```python
from build123d import *

# Parameters (mm, degrees)
SKETCH1_W           = 25
SKETCH1_H           = 30
SKETCH1_R           = 1.5
BOSS_EXTRUDE1_DEPTH = 2
BOSS_EXTRUDE2_DEPTH = 75
FILLET1_R           = 1
SKETCH3_R           = 2.25
SKETCH3_W           = 0.5
SKETCH3_H           = 6.8
CUT_EXTRUDE1_DEPTH  = 75
SKETCH5_W           = 1
SKETCH5_H           = 6.8
BOSS_EXTRUDE3_DEPTH = 2
FILLET2_R           = 10
BOSS_EXTRUDE4_DEPTH = 2


with BuildPart() as part:
    # Sketch1 → Boss-Extrude1 (new body)
    with BuildSketch(Plane(origin=(0, 0, 0), x_dir=(1, 0, 0), z_dir=(0, 1, 0))):
        with Locations((12.5, 15)):
            Rectangle(SKETCH1_W, SKETCH1_H)
        with Locations(Location((10, 22.5, 0), (0, 0, 270))):
            Circle(SKETCH1_R, mode=Mode.SUBTRACT)
        with Locations(Location((10, 7.5, 0), (0, 0, 270))):
            Circle(SKETCH1_R, mode=Mode.SUBTRACT)
    extrude(amount=BOSS_EXTRUDE1_DEPTH)

    # Sketch2 → Boss-Extrude2 (add)
    with BuildSketch(Plane(origin=(0, 2, 0), x_dir=(1, 0, 0), z_dir=(0, 1, 0))):
        Polygon((25, 30), (24, 30), (24, 0), (25, 0), (26, 0), (26, 30), align=None)
    extrude(amount=-BOSS_EXTRUDE2_DEPTH)

    # Fillet1
    fillet1_edges = [part.edges().sort_by_distance(p)[0] for p in [
        (26, 2, -15),
        (24, 0, -15),
    ]]
    fillet(fillet1_edges, radius=FILLET1_R)

    # Sketch3 → Cut-Extrude1 (cut)
    with BuildSketch(Plane.ZY.offset(-24)):
        with Locations((-20, -60.4)):
            Circle(SKETCH3_R)
        Polygon((-15, -56.2), (-15, -15.8), (-15.5, -15.8), (-25, -15.8), (-25, -56.2), (-15.5, -56.2), align=None)
        with Locations((-10, -60.4)):
            Circle(SKETCH3_R)
        with Locations((-15.25, -59.6)):
            Rectangle(SKETCH3_W, SKETCH3_H)
        with Locations((-14.75, -59.6)):
            Rectangle(SKETCH3_W, SKETCH3_H)
        Polygon((-14.5, -15.8), (-15, -15.8), (-15, -56.2), (-14.5, -56.2), (-5, -56.2), (-5, -15.8), align=None)
        with Locations((-10, -11.6)):
            Circle(SKETCH3_R)
        with Locations((-20, -11.6)):
            Circle(SKETCH3_R)
        with Locations((-15.25, -12.4)):
            Rectangle(SKETCH3_W, SKETCH3_H)
        with Locations((-14.75, -12.4)):
            Rectangle(SKETCH3_W, SKETCH3_H)
    extrude(amount=-CUT_EXTRUDE1_DEPTH, mode=Mode.SUBTRACT)

    # Sketch5 → Boss-Extrude3 (add)
    with BuildSketch(Plane(origin=(26, 0, 0), x_dir=(0, 0, -1), z_dir=(1, 0, 0))):
        with Locations((15, -12.4)):
            Rectangle(SKETCH5_W, SKETCH5_H)
        with Locations((15, -59.6)):
            Rectangle(SKETCH5_W, SKETCH5_H)
    extrude(amount=-BOSS_EXTRUDE3_DEPTH)

    # Fillet2
    fillet2_edges = [part.edges().sort_by_distance(p)[0] for p in [
        (25, -73, 0),
        (25, -73, -30),
        (0, 1, -30),
        (0, 1, 0),
    ]]
    fillet(fillet2_edges, radius=FILLET2_R)

    # Sketch8 → Boss-Extrude4 (add)
    with BuildSketch(Plane.XY):
        with BuildLine():
            Line((23, 0), (14, 0))
            Line((14, 0), (24, -10))
            Line((24, -10), (24, -1))
            ThreePointArc((24, -1), (23.707106781, -0.292893219), (23, 0))
        make_face()
    boss_extrude4 = extrude(amount=-BOSS_EXTRUDE4_DEPTH)

    # Mirror1: Boss-Extrude4 across plane
    add(boss_extrude4.mirror(Plane.XY.offset(-15)))


solid = part.part
```
For this review, take the finished solid that the model builds, in its own axes (mm). A direction names the side the tool comes from. Coordinates: 2 decimals unless noted, no trailing zeros. Order: outer loops, then holes, each group sorted by start corner. A loop starts at its lowest first (then second) coordinate and runs counter-clockwise, first axis right, second up. Notation, with made-up numbers: (-5.5, 34) -> (16.5, 34) arc R30 cw to (16.5, 61) -> close; hole circle Ø1 at (88.5, -30). An arc over 180 degrees is marked (long way). Use CSV: the item, a comma, the result in double quotes. Start each with the question number.
Item 1: We need section D-D, the plane z = -2.75. Give the boundary of the cut face in (x, y), then the cut area to 3 significant figures.
Item 2: We need section C-C, the plane z = -19.25. Give the boundary of the cut face in (x, y).
Item 3: We need section B-B, the plane z = -13. Give the boundary of the cut face in (x, y), then the cut area to 3 significant figures.
Item 4: We need section A-A, the plane y = -44. Give the boundary of the cut face in (x, z).
Item 5: Insertion check: pin 1 (3.5 mm diameter, centred on y = -60.4, z = -20, fed in from +X); pin 2 (3 mm diameter, centred on x = 18.5, y = -4, fed in from +Z); pin 3 (7 mm diameter, centred on y = -11.6, z = -20, fed in from -X); pin 4 (11.5 mm diameter, centred on x = 15, z = -8, fed in from -Y). Each pin has a flat end and moves straight along its axis. Give the tip position at first contact, or say it passes through.
Item 6: For faces 5 (the face through (10, 1, -24)), 6 (the face through (25, -56.2, -15)), 7 (the face through (11, 0, -15)), list the 3-axis set-ups (+Z, -Z, +X, -X, +Y, -Y) from which the entire face can be reached by the end or side of a thin tool; tool diameter is ignored.
Item 7: Wall thickness on probe 1 along Y at (x, z) = (24.85, -20); probe 2 along Y at (x, z) = (25.55, -20); probe 3 along Y at (x, z) = (8.5, -3.75): over which ranges is each line inside the solid? List them lowest first.
Item 8: Draft analysis for pull direction Z (two halves, no side actions). For faces 1 (the face through (25, -15.8, -15)), 2 (the face through (24.986, -10.924, -17.854)), 3 (the face through (24.5, -18.3, -30)), 4 (the face through (26, -35.5, -4.8)), state which applies: pulls with the +Z half, pulls with the -Z half, needs draft (parallel to the pull), parting line crosses it, or undercut.
Derived:
1,outline,"(3.11, 0) -> (23, 0) arc R1 cw to (24, -1) -> (24, -69.89) -> (26, -69.89) -> (26, 1) arc R1 ccw to (25, 2) -> (3.11, 2) -> close"
1,area,"186 mm^2"
2,outline,"(0, 0) -> (23, 0) arc R1 cw to (24, -1) -> (24, -9.48) -> (26, -9.48) -> (26, 1) arc R1 ccw to (25, 2) -> (0, 2) -> close; (24, -73) -> (26, -73) -> (26, -62.52) -> (24, -62.52) -> close; (24, -58.28) -> (26, -58.28) -> (26, -56.2) -> (24, -56.2) -> close; (24, -15.8) -> (26, -15.8) -> (26, -13.72) -> (24, -13.72) -> close"
3,outline,"(0, 0) -> (23, 0) arc R1 cw to (24, -1) -> (24, -15.8) -> (26, -15.8) -> (26, 1) arc R1 ccw to (25, 2) -> (0, 2) -> close; (24, -73) -> (26, -73) -> (26, -56.2) -> (24, -56.2) -> close"
3,area,"117 mm^2"
4,outline,"(24, -30) -> (26, -30) -> (26, -25) -> (24, -25) -> close; (24, -5) -> (26, -5) -> (26, 0) -> (24, 0) -> close"
5,pin 1,"passes through"
5,pin 2,"stops at z = 0"
5,pin 3,"stops at x = 24"
5,pin 4,"stops at y = 0"
6,face 5,"+Y, -Y"
6,face 6,"+X, -X"
6,face 7,"-X, -Y"
7,probe 1,"y = -73 to -62.65, -58.15 to -56.2, -15.8 to -13.85, -9.35 to 2"
7,probe 2,"y = -73 to -62.65, -58.15 to -56.2, -15.8 to -13.85, -9.35 to 1.84"
7,probe 3,"y = 0 to 2"
8,face 1,"undercut"
8,face 2,"undercut"
8,face 3,"pulls with the -Z half"
8,face 4,"needs draft"
